Input: part model. Units: mm. Frame: model coordinates. A direction names the side the tool comes from. Round coordinates to 2 decimals unless told otherwise and drop trailing zeros. Write each loop counter-clockwise with the first axis right and the second up, starting at its lowest first coordinate (ties: lowest second). Pieces come first, ordered by that corner, then holes. Notation, with made-up numbers: (39, 59) - (94, 59) arc R16 ccw to (94, 88) - close; hole circle Ø8 at (71, 41). An arc over 180 degrees is marked (long way). One line per item, written item: value. Start each with the question number.
```python
from build123d import *

# Parameters (mm, degrees)
F0_W      = 18
F0_H      = 18
F1_DEPTH  = 15
F5_DEPTH  = 11
F6_R      = 2.75
F7_DEPTH  = 15.001
F8_R      = 2
F9_W      = 11.5
F9_H      = 11
F9_W_2    = 10.9
F9_H_2    = 10.4
F10_DEPTH = 3


with BuildPart() as f1:
    # F0 (on Front) → F1 (new body)
    with BuildSketch(Plane.XZ):
        Rectangle(F0_W, F0_H)
    extrude(amount=F1_DEPTH)

    # F3 (on offset) → F5 (cut, through all)
    with BuildSketch(Plane.XZ.offset(13)):
        Polygon((5.75, -3.319764), (5.75, 3.319764), (5.75, 9.680236), (-5.75, 9.680236), (-5.75, 3.680236), (-5.75, -3.319764), (0, -6.639528), align=None)
    extrude(amount=-F5_DEPTH, mode=Mode.SUBTRACT)

    # F6 (on face) → F7 (cut, through all)
    with BuildSketch(Plane.XZ.offset(15)):
        Circle(F6_R)
    extrude(amount=-F7_DEPTH, mode=Mode.SUBTRACT)

    # F8
    f8_edges = [f1.edges().sort_by_distance(p)[0] for p in [
        (-9, -7.5, 9),
        (-9, -7.5, -9),
        (-9, 0, 0),
        (-9, -15, 0),
        (9, -7.5, -9),
        (9, -7.5, 9),
        (9, 0, 0),
        (9, -15, 0),
        (0, 0, -9),
        (0, -15, -9),
    ]]
    fillet(f8_edges, radius=F8_R)

    # F9 (on face) → F10 (join)
    with BuildSketch(Plane.XY.offset(9)):
        with Locations((0, -7.5)):
            Rectangle(F9_W, F9_H)
        with Locations((0, -7.5)):
            Rectangle(F9_W_2, F9_H_2, mode=Mode.SUBTRACT)
    extrude(amount=-F10_DEPTH)


solid = f1.part
```
Q1. Cut plane A-A, the plane z = 0. Output: boundary loops of the cut face in (x, y), and give its area (3 significant figures).
Q2. Cut plane B-B, the plane x = -2.5. Output: boundary loops of the cut face in (y, z), and give its area (3 significant figures).
Q3. Contact query for flat-ended pins moving along their axis: pin 1 Ø1.5 at (y, z) = (-10, 8) entering from -X; pin 2 Ø1.5 at (y, z) = (-5.5, 8) entering from +X. Output: stop coordinate, or through.
Q4. Cut plane D-D, the plane y = -12.25. Output: boundary loops of the cut face in (x, z), and give its area (3 significant figures).
Q5. Access query for faces 1 (the cylindrical face through (-8.43, -14.4, 1.11)), 2 (the flat face through (5.45, -8, 8)), 3 (the flat face through (5.75, -8, 1)). Directions: +Z, -Z, +X, -X, +Y, -Y. A direction counts if a zero-diameter tool reaches every point of the face in a straight line with its end or side. Return the directions, or none.
Q6. Pull-direction query (Y, two-part tool) for faces 4 (the cylindrical face through (0.1, -0.6, -8.43)), 5 (the flat face through (2.835, -7.577, -5.003)), 6 (the cylindrical face through (-0.596, -1.014, -2.685)), 7 (the flat face through (0, -2.3, 8)); classes: pulls with the +Y half, pulls with the -Y half, needs draft (parallel to the pull), parting line crosses it, or undercut.
Q7. Cut plane C-C, the plane z = 4.5. Output: boundary loops of the cut face in (x, y).
Q8. Material intervals for probe 1 along X at (y, z) = (-6, -2.5); probe 2 along Y at (x, z) = (-2, 2.5); probe 3 along Y at (x, z) = (-1.75, 8.75), sorted ascending. Write a range as from..to.
A:
1. outline: (-9, -13) arc R2 ccw to (-7, -15) - (-2.75, -15) - (-2.75, -13) - (-5.75, -13) - (-5.75, -2) - (-2.75, -2) - (-2.75, 0) - (-7, 0) arc R2 ccw to (-9, -2) - close; (2.75, -15) - (7, -15) arc R2 ccw to (9, -13) - (9, -2) arc R2 ccw to (7, 0) - (2.75, 0) - (2.75, -2) - (5.75, -2) - (5.75, -13) - (2.75, -13) - close
1. area: 118 mm²
2. outline: (-15, -7) arc R2 ccw to (-13, -9) - (-2, -9) arc R2 ccw to (0, -7) - (0, -1.15) - (-2, -1.15) - (-2, -5.2) - (-13, -5.2) - (-13, -1.15) - (-15, -1.15) - close; (-15, 1.15) - (-13, 1.15) - (-13, 6) - (-12.7, 6) - (-12.7, 9) - (-15, 9) - close; (-2.3, 6) - (-2, 6) - (-2, 1.15) - (0, 1.15) - (0, 9) - (-2.3, 9) - close
2. area: 105 mm²
3. pin 1: stops at x = -8.98
3. pin 2: stops at x = 8.98
4. outline: (-9, -7) arc R2 ccw to (-7, -9) - (7, -9) arc R2 ccw to (9, -7) - (9, 7) arc R2 ccw to (7, 9) - (5.45, 9) - (5.45, 6) - (5.75, 6) - (5.75, -3.32) - (0, -6.64) - (-5.75, -3.32) - (-5.75, 6) - (-5.45, 6) - (-5.45, 9) - (-7, 9) arc R2 ccw to (-9, 7) - close
4. area: 162 mm²
5. face 1: +Z, -Z, -X, -Y
5. face 2: +Z
5. face 3: none
6. face 4: pulls with the +Y half
6. face 5: undercut
6. face 6: needs draft
6. face 7: undercut
7. outline: (-9, -13) arc R2 ccw to (-7, -15) - (7, -15) arc R2 ccw to (9, -13) - (9, -2) arc R2 ccw to (7, 0) - (-7, 0) arc R2 ccw to (-9, -2) - close; hole (-5.75, -13) - (5.75, -13) - (5.75, -2) - (-5.75, -2) - close
8. probe 1: x = -9..-5.75, 5.75..9
8. probe 2: y = -15..-13, -2..0
8. probe 3: y = -15..-12.7, -2.3..0
